Could you check a few things on this model? Use its own coordinates, in mm. Face numbers are marked on the shaded views. A direction names the side the tool comes from. Coordinates: 2 decimals unless noted, no trailing zeros. Loops run counter-clockwise (first coordinate to the right, second up) from the corner with the lowest first, then second, coordinate; pieces in that order, holes last. Notation, with made-up numbers: (41.25, 19.5) - (47.25, 19.5) arc R23 ccw to (47.25, 36.5) - close; hole circle Ø11 at (52.5, 8.25). An arc over 180 degrees is marked (long way). One line per question, with ' | ' between items. Start each with the question number.
1. I want a section at C-C, the plane x = 21.5. Write out the boundary of the cut face in (y, z), then the cut area to 3 significant figures.
2. Please list where these lines run through material, in increasing order: L1, parallel to X at y = 3.4, z = 19; L2, parallel to Z at x = 21.5, y = 2.1. Write a range as [from, to].
3. Which directions (+Z, -Z, +X, -X, +Y, -Y) give clear straight access to the entire face, cutting with the end or side of a thin tool? Please do the marked faces 3 and 4.
4. I want a section at A-A, the plane y = 1.15. Write out the boundary of the cut face in (x, z) (1 decimal), then the cut area to 3 significant figures.
5. We'd pull the mould along X, two halves only. Please class the marked faces 1 and 2: pulls with the +X half, pulls with the -X half, needs draft (parallel to the pull), parting line crosses it, or undercut.
6. I'm going to push flat-ended pins straight in: P1, Ø1, axis at x = 14, z = 13.5, coming from the -Y side; P2, Ø2.5, axis at x = 21.5, z = 19, coming from the +Y side. Where does each tip first touch, or does it pass through?
7. I want a section at D-D, the plane z = 0. Write out the boundary of the cut face in (x, y).
8. I want a section at B-B, the plane z = -19. Write out the boundary of the cut face in (x, y), then the cut area to 3 significant figures.
from build123d import *

# Parameters (mm, degrees)
SKETCH1_W           = 50
SKETCH1_H           = 45
SKETCH1_R           = 1.5625
BOSS_EXTRUDE1_DEPTH = 4.7625
FILLET1_R           = 2
CUT_EXTRUDE1_DEPTH  = 5.7625


with BuildPart() as part:
    # Sketch1 → Boss-Extrude1 (new body)
    with BuildSketch(Plane(origin=(0, 0, 0), x_dir=(1, 0, 0), z_dir=(0, 1, 0))):
        Rectangle(SKETCH1_W, SKETCH1_H)
        with Locations((-21.5, 19)):
            Circle(SKETCH1_R, mode=Mode.SUBTRACT)
        with Locations((21.5, 19)):
            Circle(SKETCH1_R, mode=Mode.SUBTRACT)
        with Locations((21.5, -19)):
            Circle(SKETCH1_R, mode=Mode.SUBTRACT)
        with Locations((-21.5, -19)):
            Circle(SKETCH1_R, mode=Mode.SUBTRACT)
    extrude(amount=BOSS_EXTRUDE1_DEPTH)

    # Fillet1
    fillet1_edges = [part.edges().sort_by_distance(p)[0] for p in [
        (-25, 2.38125, -22.5),
        (25, 2.38125, -22.5),
        (25, 2.38125, 22.5),
        (-25, 2.38125, 22.5),
    ]]
    fillet(fillet1_edges, radius=FILLET1_R)

    # Sketch2 → Cut-Extrude1 (cut, through all)
    with BuildSketch(Plane(origin=(0, 4.7625, 0), x_dir=(1, 0, 0), z_dir=(0, 1, 0))):
        with BuildLine():
            Line((-25, 5.6), (-19, 5.6))
            Line((-19, 5.6), (-19, -3))
            Line((-19, -3), (-20, -3))
            ThreePointArc((-20, -3), (-23, 0), (-20, 3))
            Line((-20, 3), (-20.1, 4.5))
            Line((-20.1, 4.5), (-25, 4.5))
            Line((-25, 4.5), (-25, 5.6))
        make_face()
    cut_extrude1 = extrude(amount=-CUT_EXTRUDE1_DEPTH, mode=Mode.SUBTRACT)

    # Mirror1: Cut-Extrude1 across plane
    add(cut_extrude1.mirror(Plane(origin=(0, 0, 0), x_dir=(0, 0, 1), z_dir=(1, 0, 0))), mode=Mode.SUBTRACT)


solid = part.part
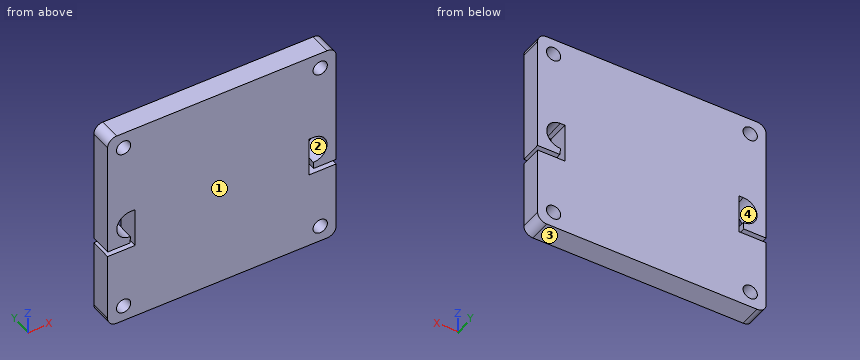
Results are:
1) outline: (0, -22.5) - (4.76, -22.5) - (4.76, -20.56) - (0, -20.56) - close; (0, -17.44) - (4.76, -17.44) - (4.76, -5.6) - (0, -5.6) - close; (0, -4.5) - (4.76, -4.5) - (4.76, -2.6) - (0, -2.6) - close; (0, 2.6) - (4.76, 2.6) - (4.76, 17.44) - (0, 17.44) - close; (0, 20.56) - (4.76, 20.56) - (4.76, 22.5) - (0, 22.5) - close | area: 155 mm2
2) L1: x = [-25, -23.06], [-19.94, 19.94], [23.06, 25] | L2: z = [-22.5, -20.56], [-17.44, -5.6], [-4.5, -2.6], [2.6, 17.44], [20.56, 22.5]
3) face 3: -Z, +X, -X, +Y, -Y | face 4: +Y, -Y
4) outline: (-25, -20.5) arc R2 ccw to (-23, -22.5) - (23, -22.5) arc R2 ccw to (25, -20.5) - (25, -5.6) - (19, -5.6) - (19, 3) - (20, 3) arc R3 cw to (20, -3) - (20.1, -4.5) - (25, -4.5) - (25, 20.5) arc R2 ccw to (23, 22.5) - (-23, 22.5) arc R2 ccw to (-25, 20.5) - (-25, -4.5) - (-20.1, -4.5) - (-20, -3) arc R3 cw to (-20, 3) - (-19, 3) - (-19, -5.6) - (-25, -5.6) - close; hole circle Ø3.1 at (-21.5, -19); hole circle Ø3.1 at (-21.5, 19); hole circle Ø3.1 at (21.5, -19); hole circle Ø3.1 at (21.5, 19) | area: 2,160 mm2
5) face 1: needs draft | face 2: undercut
6) P1: stops at y = 0 | P2: passes through
7) outline: (-25, 0) - (-23, 0) - (-23, 4.76) - (-25, 4.76) - close; (-19, 0) - (19, 0) - (19, 4.76) - (-19, 4.76) - close; (23, 0) - (25, 0) - (25, 4.76) - (23, 4.76) - close
8) outline: (-25, 0) - (-23.06, 0) - (-23.06, 4.76) - (-25, 4.76) - close; (-19.94, 0) - (19.94, 0) - (19.94, 4.76) - (-19.94, 4.76) - close; (23.06, 0) - (25, 0) - (25, 4.76) - (23.06, 4.76) - close | area: 208 mm2
